Build history of the part. All positions in model axes, mm. A direction names the side the tool comes from. Coordinates: 2 decimals unless noted, no trailing zeros. Order: outer loops, then holes, each group sorted by start corner. A loop starts at its lowest first (then second) coordinate and runs counter-clockwise, first axis right, second up. Notation, with made-up numbers: (36.25, -7) - (80.25, -7) arc R17 cw to (80.25, 16) - close; hole circle Ø8 at (34.5, 31.25). An arc over 180 degrees is marked (long way). One line per item, written item: value.
from build123d import *

# Parameters (mm, degrees)
SKETCH_1_R          = 9.5
EXTRUDE_1_DEPTH     = 6
EXTRUDE_1_TAPER     = 5
SKETCH_2_R          = 8
SKETCH_2_R_2        = 4.5
CUT_EXTRUDE_2_DEPTH = 3
SKETCH_3_R          = 3.5
CUT_EXTRUDE_3_DEPTH = 4
SKETCH_4_R          = 3.55
SKETCH_4_R_2        = 3
EXTRUDE_2_DEPTH     = 2
FILLET_1_R          = 0.5


with BuildPart() as part:
    # Эскиз1 → Бобышка-Вытянуть1 (new body)
    with BuildSketch(Plane.XY):
        Circle(SKETCH_1_R)
    extrude(amount=EXTRUDE_1_DEPTH, taper=EXTRUDE_1_TAPER)

    # Эскиз2 → Вырез-Вытянуть2 (cut)
    with BuildSketch(Plane(origin=(0, 0, 0), x_dir=(-1, 0, 0), z_dir=(0, 0, -1))):
        Circle(SKETCH_2_R)
        Circle(SKETCH_2_R_2, mode=Mode.SUBTRACT)
    extrude(amount=-CUT_EXTRUDE_2_DEPTH, mode=Mode.SUBTRACT)

    # Эскиз3 → Вырез-Вытянуть3 (cut)
    with BuildSketch(Plane.XY.offset(6)):
        Circle(SKETCH_3_R)
    extrude(amount=-CUT_EXTRUDE_3_DEPTH, mode=Mode.SUBTRACT)

    # Эскиз4 → Бобышка-Вытянуть2 (add)
    with BuildSketch(Plane.XY.offset(6)):
        Circle(SKETCH_4_R)
        Circle(SKETCH_4_R_2, mode=Mode.SUBTRACT)
    extrude(amount=-EXTRUDE_2_DEPTH)

    # Скругление1
    fillet_1_edges = [part.edges().sort_by_distance(p)[0] for p in [
        (-8.975068019, 0, 6),
    ]]
    fillet(fillet_1_edges, radius=FILLET_1_R)


solid = part.part
1. Band-saw the part on C-C, the plane z = 2.35. Give the cut face in (x, y).
Values found:
outline: circle Ø18.59 at (0, 0); circle Ø9 at (0, 0); hole circle Ø16 at (0, 0); hole circle Ø7 at (0, 0)
2. Probe line 1 along Y through (x, z) = (0, 2.3); line 2 along X through (y, z) = (3, 1.5); line 3 along X through (y, z) = (6.5, 0.9). List the from-to ranges inside material, lowest first.
Values found:
line 1: y = -9.3 to -8, -4.5 to -3.5, 3.5 to 4.5, 8 to 9.3
line 2: x = -8.88 to -7.42, -3.35 to 3.35, 7.42 to 8.88
line 3: x = -6.82 to -4.66, 4.66 to 6.82
3. Flat gauge pins, fed straight in: P1, Ø3, axis at x = -3, z = 2.5, coming from the +Y side; P2, Ø1.5, axis at y = -7.5, z = 5.5, coming from the -X side; P3, Ø3, axis at x = -0.5, z = 1.5, coming from the -Y side. Where does each tip first touch, or does it go through?
Values found:
P1: stops at y = 9.19
P2: stops at x = -5.99
P3: stops at y = -9.5
4. 3-axis set-ups, long thin cutter, end or side, ignore diameter. For faces 1 (the face through (1.73, -7.81, 1.48)), 2 (the face through (4, 0, 6)), 3 (the face through (3, 1, 4)): which of +Z, -Z, +X, -X, +Y, -Y reach the whole face in a straight line?
Values found:
face 1: -Z
face 2: +Z, +X, -X, +Y, -Y
face 3: none
5. Band-saw the part on D-D, the plane z = 4.3. Give the cut face in (x, y).
Values found:
outline: circle Ø18.25 at (0, 0); hole circle Ø6 at (0, 0)
6. Two-plate mould, pull along Y, no slides. Class faces 4 (the face through (-3, 0, 5)), 5 (the face through (0, 0, 0)), 6 (the face through (-9.19, 0.4, 3.43)): pulls with the +Y half, pulls with the -Y half, needs draft (parallel to the pull), parting line crosses it, or undercut.
Values found:
face 4: undercut
face 5: needs draft
face 6: parting line crosses it
7. Band-saw the part on A-A, the plane x = 0. Give the cut face in (y, z) (3 decimals).
Values found:
outline: (-9.5, 0) - (-8, 0) - (-8, 3) - (-4.5, 3) - (-4.5, 0) - (4.5, 0) - (4.5, 3) - (8, 3) - (8, 0) - (9.5, 0) - (9.015, 5.544) arc R0.5 ccw to (8.517, 6) - (3, 6) - (3, 4) - (3.5, 4) - (3.5, 2) - (-3.5, 2) - (-3.5, 4) - (-3, 4) - (-3, 6) - (-8.517, 6) arc R0.5 ccw to (-9.015, 5.544) - close
